Build history of the part. All positions in model axes, mm. A direction names the side the tool comes from. Round coordinates to 2 decimals unless told otherwise and drop trailing zeros. Write each loop counter-clockwise with the first axis right and the second up, starting at its lowest first coordinate (ties: lowest second). Pieces come first, ordered by that corner, then holes. Notation, with made-up numbers: M 56.25,-35.75 L 101.25,-35.75 A12 ccw 101.25,-22.75 Z; hole C 77.25,37 d4. An arc over 180 degrees is marked long. Write item = value, one per line.
from build123d import *

# Parameters (mm, degrees)
F1_DEPTH = 38.1
F2_W     = 12.7
F2_H     = 12.000482
F2_H_2   = 13.399518
F3_DEPTH = 6.35


with BuildPart() as f1:
    # F0 (on Front) → F1 (new body)
    with BuildSketch(Plane.XZ):
        Polygon((0, 12.7), (0, 0), (25.4, 0), (25.4, 31.75), (12.7, 31.75), (12.7, 12.7), align=None)
    extrude(amount=F1_DEPTH)

    # F2 (on face) → F3 (join)
    with BuildSketch(Plane.XY.offset(31.75)):
        with Locations((19.05, -32.099759)):
            Rectangle(F2_W, F2_H)
        with Locations((19.05, -6.699759)):
            Rectangle(F2_W, F2_H_2)
    extrude(amount=F3_DEPTH)


solid = f1.part
1. Mould opens along Y. For faces 1 (the face through (13, -19, 0)), 2 (the face through (15, 0, 15)), 3 (the face through (15, -38.1, 15)), 4 (the face through (19, -13.4, 35)) say: pulls with the +Y half, pulls with the -Y half, needs draft (parallel to the pull), parting line crosses it, or undercut.
Responses:
face_1 = needs draft
face_2 = pulls with the +Y half
face_3 = pulls with the -Y half
face_4 = undercut
2. Band-saw the part on A-A (x = 22.25). List the corners of the cut face in (y, z), plus the area to 3 significant figures.
Responses:
outline = M -38.1,0 L 0,0 L 0,38.1 L -13.4,38.1 L -13.4,31.75 L -26.1,31.75 L -26.1,38.1 L -38.1,38.1 Z
area = 1,370 mm²
3. Tool access for faces 5 (the face through (19, -20, 31.75)), 6 (the face through (0, -19, 6)), 7 (the face through (6, -19, 12.7)): list every direction of +Z, -Z, +X, -X, +Y, -Y with a clear straight run to the whole face (end or side of a thin tool).
Responses:
face_5 = +Z, +X, -X
face_6 = +Z, -Z, -X, +Y, -Y
face_7 = +Z, -X, +Y, -Y
4. Flat gauge pins, fed straight in: pin 1 (6.5 mm diameter, centred on x = 9, y = -23, fed in from +Z); pin 2 (4 mm diameter, centred on y = -34, z = 16.5, fed in from -X). Where does each tip first touch, or does it go through?
Responses:
pin_1 = 12.7
pin_2 = 12.7
5. Band-saw the part on B-B (y = -17.5). List the corners of the cut face in (x, z), plus the area to 3 significant figures.
Responses:
outline = M 0,0 L 25.4,0 L 25.4,31.75 L 12.7,31.75 L 12.7,12.7 L 0,12.7 Z
area = 565 mm²
6. Band-saw the part on C-C (z = 15.5). List the corners of the cut face in (x, y), plus the area to 3 significant figures.
Responses:
outline = M 12.7,-38.1 L 25.4,-38.1 L 25.4,0 L 12.7,0 Z
area = 484 mm²
7. Band-saw the part on D-D (y = -8). List the corners of the cut face in (x, z).
Responses:
outline = M 0,0 L 25.4,0 L 25.4,38.1 L 12.7,38.1 L 12.7,12.7 L 0,12.7 Z
8. Probe probe 1 along Z at (x, y) = (21.5, -14); probe 2 along X at (y, z) = (-7.5, 36); probe 3 along Z at (x, y) = (1.5, -35.5). List the from-to ranges inside material, lowest first.
Responses:
probe_1 = 0 to 31.75
probe_2 = 12.7 to 25.4
probe_3 = 0 to 12.7
